```python
from build123d import *

# Parameters (mm, degrees)
F1_DEPTH = 165.1
F0_W     = 19.05
F0_H     = 69.85
F0_R     = 9.525
F2_DEPTH = 95.25
F3_DEPTH = 107.95
F4_R     = 9.525
F5_DEPTH = 107.95
F6_DEPTH = 76.2
F7_DEPTH = 101.6
F8_R     = 6.35
F9_DEPTH = 95.251


with BuildPart() as f1:
    # F0 (on Front) → F1 (new body, symmetric)
    with BuildSketch(Plane.XZ):
        Polygon((-76.2, 25.4), (-95.25, 25.4), (-95.25, 0), (95.25, 0), (95.25, 25.4), (76.2, 25.4), (25.4, 25.4), (-25.4, 25.4), align=None)
    extrude(amount=F1_DEPTH, both=True)

    # F0 (on Front) → F2 (join, symmetric)
    with BuildSketch(Plane.XZ):
        with Locations((-85.725, 60.325)):
            Rectangle(F0_W, F0_H)
        with BuildLine():
            Line((-76.2, 95.25), (-76.2, 25.4))
            Line((-76.2, 25.4), (-25.4, 25.4))
            Line((-25.4, 25.4), (-25.4, 69.85))
            ThreePointArc((-25.4, 69.85), (-17.9605122421, 87.8105122421), (0, 95.25))
            Line((0, 95.25), (-76.2, 95.25))
        make_face()
        with BuildLine():
            Line((-25.4, 69.85), (-25.4, 25.4))
            Line((-25.4, 25.4), (25.4, 25.4))
            Line((25.4, 25.4), (25.4, 69.85))
            ThreePointArc((25.4, 69.85), (17.9605122421, 87.8105122421), (0, 95.25))
            ThreePointArc((0, 95.25), (-17.9605122421, 87.8105122421), (-25.4, 69.85))
        make_face()
        with Locations((0, 69.85)):
            Circle(F0_R, mode=Mode.SUBTRACT)
        with BuildLine():
            Line((25.4, 69.85), (25.4, 25.4))
            Line((25.4, 25.4), (76.2, 25.4))
            Line((76.2, 25.4), (76.2, 95.25))
            Line((76.2, 95.25), (0, 95.25))
            ThreePointArc((0, 95.25), (17.9605122421, 87.8105122421), (25.4, 69.85))
        make_face()
        with Locations((85.725, 60.325)):
            Rectangle(F0_W, F0_H)
    extrude(amount=F2_DEPTH, both=True)

    # F0 (on Front) → F3 (join, symmetric)
    with BuildSketch(Plane.XZ):
        with BuildLine():
            Line((-25.4, 69.85), (-25.4, 25.4))
            Line((-25.4, 25.4), (25.4, 25.4))
            Line((25.4, 25.4), (25.4, 69.85))
            ThreePointArc((25.4, 69.85), (17.9605122421, 87.8105122421), (0, 95.25))
            ThreePointArc((0, 95.25), (-17.9605122421, 87.8105122421), (-25.4, 69.85))
        make_face()
        with Locations((0, 69.85)):
            Circle(F0_R, mode=Mode.SUBTRACT)
    extrude(amount=F3_DEPTH, both=True)

    # F4 (on Right) → F5 (join, symmetric)
    with BuildSketch(Plane.YZ):
        with BuildLine():
            Line((25.4, 0), (25.4, 69.85))
            ThreePointArc((25.4, 69.85), (0, 95.25), (-25.4, 69.85))
            Line((-25.4, 69.85), (-25.4, 0))
            Line((-25.4, 0), (25.4, 0))
        make_face()
        with Locations((0, 69.85)):
            Circle(F4_R, mode=Mode.SUBTRACT)
    extrude(amount=F5_DEPTH, both=True)

    # F0 (on Front) → F6 (cut, symmetric)
    with BuildSketch(Plane.XZ):
        with BuildLine():
            Line((-76.2, 95.25), (-76.2, 25.4))
            Line((-76.2, 25.4), (-25.4, 25.4))
            Line((-25.4, 25.4), (-25.4, 69.85))
            ThreePointArc((-25.4, 69.85), (-17.9605122421, 87.8105122421), (0, 95.25))
            Line((0, 95.25), (-76.2, 95.25))
        make_face()
        with BuildLine():
            Line((-25.4, 69.85), (-25.4, 25.4))
            Line((-25.4, 25.4), (25.4, 25.4))
            Line((25.4, 25.4), (25.4, 69.85))
            ThreePointArc((25.4, 69.85), (17.9605122421, 87.8105122421), (0, 95.25))
            ThreePointArc((0, 95.25), (-17.9605122421, 87.8105122421), (-25.4, 69.85))
        make_face()
        with Locations((0, 69.85)):
            Circle(F0_R, mode=Mode.SUBTRACT)
        with BuildLine():
            Line((25.4, 69.85), (25.4, 25.4))
            Line((25.4, 25.4), (76.2, 25.4))
            Line((76.2, 25.4), (76.2, 95.25))
            Line((76.2, 95.25), (0, 95.25))
            ThreePointArc((0, 95.25), (17.9605122421, 87.8105122421), (25.4, 69.85))
        make_face()
        with Locations((0, 69.85)):
            Circle(F0_R)
    extrude(amount=F6_DEPTH, both=True, mode=Mode.SUBTRACT)

    # F4 (on Right) → F7 (cut, symmetric)
    with BuildSketch(Plane.YZ):
        with Locations((0, 69.85)):
            Circle(F4_R)
    extrude(amount=F7_DEPTH, both=True, mode=Mode.SUBTRACT)

    # F8 (on face) → F9 (cut, through all)
    with BuildSketch(Plane(origin=(0, 0, 0), x_dir=(1, 0, 0), z_dir=(0, 0, -1))):
        with Locations((-57.15, 139.7)):
            Circle(F8_R)
        with Locations((57.15, 139.7)):
            Circle(F8_R)
        with Locations((57.15, -139.7)):
            Circle(F8_R)
        with Locations((-57.15, -139.7)):
            Circle(F8_R)
    extrude(amount=-F9_DEPTH, mode=Mode.SUBTRACT)


solid = f1.part
```
Work out the finished part from the listing and answer in its coordinate system (mm). A direction names the side the tool comes from. Round coordinates to 2 decimals unless told otherwise and drop trailing zeros. Loops run counter-clockwise (first coordinate to the right, second up) from the corner with the lowest first, then second, coordinate; pieces in that order, holes last.
(1) The part is cut by section B-B, the plane y = -139.7. Give the vertices of the cut face in (x, z), and give its area (3 significant figures).
Computed values:
outline: (-95.25, 0) - (-63.5, 0) - (-63.5, 25.4) - (-95.25, 25.4) - close; (-50.8, 0) - (50.8, 0) - (50.8, 25.4) - (-50.8, 25.4) - close; (63.5, 0) - (95.25, 0) - (95.25, 25.4) - (63.5, 25.4) - close
area: 4,190 mm2
(2) The part is cut by section D-D, the plane y = -99. Give the vertices of the cut face in (x, z) (3 decimals), and give its area (3 significant figures).
Computed values:
outline: (-95.25, 0) - (95.25, 0) - (95.25, 25.4) - (25.4, 25.4) - (25.4, 69.85) arc R25.4 ccw to (-25.4, 69.85) - (-25.4, 25.4) - (-95.25, 25.4) - close; hole circle Ø19.05 at (0, 69.85)
area: 7,830 mm2
(3) The mould has two halves that part along X. Classify faces 6 (the flat face through (-76.2, -1, 53)), 7 (the flat face through (-25.4, 102, 48)), 8 (the flat face through (-1, -165.1, 13)), 9 (the cylindrical face through (-7.02, 91.85, 76.29)): pulls with the +X half, pulls with the -X half, needs draft (parallel to the pull), parting line crosses it, or undercut.
Computed values:
face 6: undercut
face 7: pulls with the -X half
face 8: needs draft
face 9: undercut
(4) For faces 1 (the flat face through (102, 25.4, 34)), 2 (the flat face through (25.4, -102, 47)), 3 (the flat face through (-59, -95.25, 61)), 4 (the cylindrical face through (101.689, 0.559, 95.244)), 5 (the flat face through (0, -107.95, 53)), determine the directions among +Z, -Z, +X, -X, +Y, -Y from which every point of the face is accessible in a straight line to the end or side of a thin tool.
Computed values:
face 1: +Z, -Z, +X, +Y
face 2: +Z, +X, -Y
face 3: +Z, -X, -Y
face 4: +Z, +X
face 5: +Z, +X, -X, -Y
(5) Find the intervals of material crossed by L1, parallel to Y at x = -57.15, z = 8.5; L2, parallel to Y at x = -64.5, z = 81.5; L3, parallel to Z at x = -105, y = 0 (3 decimals), in increasing order.
Computed values:
L1: y = -165.1 to -146.05, -133.35 to 133.35, 146.05 to 165.1
L2: y = -95.25 to -76.2, 76.2 to 95.25
L3: z = 0 to 60.325, 79.375 to 95.25
(6) The part is cut by section C-C, the plane z = 22. Give the vertices of the cut face in (x, y).
Computed values:
outline: (-107.95, -25.4) - (-95.25, -25.4) - (-95.25, -165.1) - (95.25, -165.1) - (95.25, -25.4) - (107.95, -25.4) - (107.95, 25.4) - (95.25, 25.4) - (95.25, 165.1) - (-95.25, 165.1) - (-95.25, 25.4) - (-107.95, 25.4) - close; hole circle Ø12.7 at (-57.15, -139.7); hole circle Ø12.7 at (-57.15, 139.7); hole circle Ø12.7 at (57.15, -139.7); hole circle Ø12.7 at (57.15, 139.7)
(7) Each of these flat-tipped pins is pushed along its axis until it touches: P1, Ø1.5, axis at x = 74, y = 51, coming from the -Z side; P2, Ø1, axis at x = -49.5, z = 63, coming from the +Y side; P3, Ø1, axis at y = -83, z = 42, coming from the +X side; P4, Ø1, axis at y = -23.5, z = 84, coming from the -X side. Where does it stop, or does it pass through?
Computed values:
P1: stops at z = 0
P2: stops at y = 95.25
P3: stops at x = 95.25
P4: stops at x = -95.25
(8) The part is cut by section A-A, the plane x = -89.5. Give the vertices of the cut face in (y, z) (3 decimals), and give its area (3 significant figures).
Computed values:
outline: (-165.1, 0) - (165.1, 0) - (165.1, 25.4) - (95.25, 25.4) - (95.25, 95.25) - (-95.25, 95.25) - (-95.25, 25.4) - (-165.1, 25.4) - close; hole circle Ø19.05 at (0, 69.85)
area: 21,400 mm2
